Verification items for the finished model (mm, model axes). A direction names the side the tool comes from. Coordinates: 2 decimals unless noted, no trailing zeros. Order: outer loops, then holes, each group sorted by start corner. A loop starts at its lowest first (then second) coordinate and runs counter-clockwise, first axis right, second up. Notation, with made-up numbers: (-19, 71.5) -> (15, 71.5) arc R21 ccw to (15, 84.5) -> close; hole circle Ø1 at (88, 33). An arc over 180 degrees is marked (long way). Use CSV: the item, a comma, the result in double quotes. Start each with the question number.
1) Release check for a two-part mould opening along Y. For faces 4 (the flat face through (11, 25.4, 52)), 5 (the cylindrical face through (-3.325, 12.522, 92.19)), 6 (the flat face through (5.08, 6, 64)) record: released by +Y, released by -Y, zero draft, split by the parting line, or undercut.
2) Scan lines: line 1 along X through (y, z) = (19, 13.5); line 2 along X through (y, z) = (16.25, 36) (3 decimals); line 3 along Y through (x, z) = (8, 93). Record each from-to range of solid material in increasing order.
3) Sectioned sample at D-D on z = 12.7. Record the boundary of the cut face in (x, y), then the cut area to 3 significant figures.
4) Tool access check on faces 1 (the flat face through (13, 19, 25.4)), 2 (the flat face through (8, 5.08, 16)), 3 (the flat face through (25.4, 13, 50)). Record the directions out of +Z, -Z, +X, -X, +Y, -Y that give a thin tool (end or side, any length) a straight path to the whole face; none if there is none.
5) Sectioned sample at B-B on x = 21.5. Record the boundary of the cut face in (y, z).
6) Sectioned sample at C-C on y = 21.5. Record the boundary of the cut face in (x, z).
7) Go/stop test with flat-tipped pins: pin 1 (6 mm diameter, centred on y = 14.5, z = 68.5, fed in from -X); pin 2 (12 mm diameter, centred on x = -1, z = 29, fed in from -Y); pin 3 (1.6 mm diameter, centred on x = 7.5, y = 9, fed in from +Z); pin 4 (2.5 mm diameter, centred on y = 12.7, z = 12.7, fed in from +X). Record where each tip stops, or that it passes through.
from build123d import *

# Parameters (mm, degrees)
F0_W      = 25.4
F0_H      = 25.4
F1_DEPTH  = 101.6
F2_W      = 15.24
F2_H      = 15.24
F3_DEPTH  = 76.2
F6_START  = -3.175
F5_W      = 3.175
F5_H      = 15.24
F6_DEPTH  = 12.065
F4_R      = 2.15
F7_DEPTH  = 6.6675
F8_R      = 2.15
F9_DEPTH  = 6.6675
F10_W     = 1.27
F10_H     = 1.27
F12_DEPTH = 3.175
F11_W     = 1.27
F11_H     = 1.27
F13_DEPTH = 3.175
F14_W     = 12.7794421278
F14_H     = 4.0193349123
F15_DEPTH = 5.08
F16_W     = 25.4
F16_H     = 6.7783382893
F16_W_2   = 12.7794421278
F16_H_2   = 4.0193349123
F17_DEPTH = 5.08
F18_W     = 25.4
F18_H     = 6.7783382893
F19_DEPTH = 5.08
F20_R     = 2.15
F21_DEPTH = 5.08
F23_DEPTH = 25.4
F24_W     = 21.59
F24_H     = 1.6
F25_DEPTH = 77.47
F26_W     = 12.7794421278
F26_H     = 1.3284322977
F27_DEPTH = 5.08


with BuildPart() as f1:
    # F0 (on Top) → F1 (new body)
    with BuildSketch(Plane.XY):
        with Locations((12.7, 12.7)):
            Rectangle(F0_W, F0_H)
    extrude(amount=F1_DEPTH)

    # F2 (on face) → F3 (cut)
    with BuildSketch(Plane.XY.offset(101.6)):
        with Locations((12.7, 12.7)):
            Rectangle(F2_W, F2_H)
    extrude(amount=-F3_DEPTH, mode=Mode.SUBTRACT)

    # F5 (on face) → F6 (cut)
    with BuildSketch(Plane.XY.offset(25.4).offset(F6_START)):
        with Locations((17.145, 12.7)):
            Rectangle(F5_W, F5_H)
        with Locations((8.255, 12.7)):
            Rectangle(F5_W, F5_H)
    extrude(amount=-F6_DEPTH, mode=Mode.SUBTRACT)

    # F4 (on face) → F7 (cut, through all)
    with BuildSketch(Plane.YZ.offset(25.4)):
        with Locations((12.7, 12.7)):
            Circle(F4_R)
    extrude(amount=-F7_DEPTH, mode=Mode.SUBTRACT)

    # F8 (on face) → F9 (cut, through all)
    with BuildSketch(Plane(origin=(0, 0, 0), x_dir=(0, -1, 0), z_dir=(-1, 0, 0))):
        with Locations((-12.7, 12.7)):
            Circle(F8_R)
    extrude(amount=-F9_DEPTH, mode=Mode.SUBTRACT)

    # F10 (on face) → F12 (cut, through all)
    with BuildSketch(Plane.XY.offset(25.4)):
        with Locations((17.2085, 18.923)):
            Rectangle(F10_W, F10_H)
        with Locations((17.2085, 10.541)):
            Rectangle(F10_W, F10_H)
    extrude(amount=-F12_DEPTH, mode=Mode.SUBTRACT)

    # F11 (on face) → F13 (cut, through all)
    with BuildSketch(Plane.XY.offset(25.4)):
        with Locations((8.1467080774, 6.477)):
            Rectangle(F11_W, F11_H)
        with Locations((8.1467080774, 14.859)):
            Rectangle(F11_W, F11_H)
    extrude(amount=-F13_DEPTH, mode=Mode.SUBTRACT)

    # F14 (on face) → F15 (cut, through all)
    with BuildSketch(Plane(origin=(0, 0, 0), x_dir=(0, -1, 0), z_dir=(-1, 0, 0))):
        with Locations((-12.943365844, 98.2619002461)):
            Rectangle(F14_W, F14_H)
    extrude(amount=-F15_DEPTH, mode=Mode.SUBTRACT)

    # F16 (on face) → F17 (join)
    with BuildSketch(Plane(origin=(0, 0, 0), x_dir=(0, -1, 0), z_dir=(-1, 0, 0))):
        with Locations((-12.7, 98.2108308554)):
            Rectangle(F16_W, F16_H)
        with Locations((-12.943365844, 98.2619002461)):
            Rectangle(F16_W_2, F16_H_2, mode=Mode.SUBTRACT)
    extrude(amount=F17_DEPTH)

    # F18 (on face) → F19 (join)
    with BuildSketch(Plane(origin=(-5.08, 0, 0), x_dir=(0, -1, 0), z_dir=(-1, 0, 0))):
        with Locations((-12.7, 98.2108308554)):
            Rectangle(F18_W, F18_H)
    extrude(amount=F19_DEPTH)

    # F20 (on face) → F21 (cut)
    with BuildSketch(Plane(origin=(-10.16, 0, 0), x_dir=(0, -1, 0), z_dir=(-1, 0, 0))):
        with Locations((-12.7924755216, 98.2300043106)):
            Circle(F20_R)
    extrude(amount=-F21_DEPTH, mode=Mode.SUBTRACT)

    # F22 (on face) → F23 (join, through all)
    with BuildSketch(Plane.XZ):
        with BuildLine():
            ThreePointArc((-10.16, 94.8216617107), (-3.2465860676, 92.1186283067), (0, 85.4431986809))
            Line((0, 85.4431986809), (0, 94.8216617107))
            Line((0, 94.8216617107), (-10.16, 94.8216617107))
        make_face()
    extrude(amount=-F23_DEPTH)

    # F24 (on face) → F25 (cut)
    with BuildSketch(Plane.XY.offset(101.6)):
        with Locations((12.7, 16.93682)):
            Rectangle(F24_W, F24_H)
        with Locations((12.7, 8.57046)):
            Rectangle(F24_W, F24_H)
        with Locations((12.7, 12.75364)):
            Rectangle(F24_W, F24_H)
    extrude(amount=-F25_DEPTH, mode=Mode.SUBTRACT)

    # F26 (on face) → F27 (cut)
    with BuildSketch(Plane.YZ.offset(5.08)):
        with Locations((12.943365844, 100.9357838511)):
            Rectangle(F26_W, F26_H)
    extrude(amount=-F27_DEPTH, mode=Mode.SUBTRACT)


solid = f1.part
Answers follow:
1,face 4,"released by +Y"
1,face 5,"zero draft"
1,face 6,"undercut"
2,line 1,"x = 0 to 6.67, 9.84 to 15.56, 18.73 to 25.4"
2,line 2,"x = 0 to 1.905, 23.495 to 25.4"
2,line 3,"y = 0 to 5.08, 20.32 to 25.4"
3,outline,"(0, 0) -> (25.4, 0) -> (25.4, 10.55) -> (18.73, 10.55) -> (18.73, 5.08) -> (15.56, 5.08) -> (15.56, 20.32) -> (18.73, 20.32) -> (18.73, 14.85) -> (25.4, 14.85) -> (25.4, 25.4) -> (0, 25.4) -> (0, 14.85) -> (6.67, 14.85) -> (6.67, 20.32) -> (9.84, 20.32) -> (9.84, 5.08) -> (6.67, 5.08) -> (6.67, 10.55) -> (0, 10.55) -> close"
3,area,"491 mm²"
4,face 1,"+Z"
4,face 2,"none"
4,face 3,"+Z, -Z, +X, +Y, -Y"
5,outline,"(0, 0) -> (25.4, 0) -> (25.4, 101.6) -> (17.74, 101.6) -> (17.74, 24.13) -> (16.14, 24.13) -> (16.14, 101.6) -> (13.55, 101.6) -> (13.55, 24.13) -> (11.95, 24.13) -> (11.95, 101.6) -> (9.37, 101.6) -> (9.37, 24.13) -> (7.77, 24.13) -> (7.77, 101.6) -> (0, 101.6) -> close; hole circle Ø4.3 at (12.7, 12.7)"
6,outline,"(-10.16, 94.82) arc R10.19 cw to (0, 85.44) -> (0, 0) -> (25.4, 0) -> (25.4, 101.6) -> (-10.16, 101.6) -> close"
7,pin 1,"stops at x = 0"
7,pin 2,"stops at y = 0"
7,pin 3,"stops at z = 25.4"
7,pin 4,"stops at x = 15.56"
